from build123d import *

# Parameters (mm, degrees)
SKETCH1_R           = 60
BOSS_EXTRUDE1_DEPTH = 1500
CUT_EXTRUDE1_REACH  = 1504.398


with BuildPart() as part:
    # Sketch1 → Boss-Extrude1 (new body)
    with BuildSketch(Plane(origin=(0, 0, 0), x_dir=(1, 0, 0), z_dir=(0, 1, 0))):
        with Locations(Location((0, 0, 0), (0, 0, 270))):
            Circle(SKETCH1_R)
    extrude(amount=BOSS_EXTRUDE1_DEPTH)

    # Sketch2 → Cut-Extrude1 (cut, up to next)
    with BuildSketch(Plane(origin=(0, 1500, 0), x_dir=(1, 0, 0), z_dir=(0, 1, 0)), mode=Mode.PRIVATE) as cut_extrude1_sk1:
        Polygon((-10.998522628, 19.05), (-21.997045256, 0), (-10.998522628, -19.05), (10.998522628, -19.05), (21.997045256, 0), (10.998522628, 19.05), align=None)
    cut_extrude1_tool1 = extrude(cut_extrude1_sk1.sketch, amount=-CUT_EXTRUDE1_REACH, mode=Mode.PRIVATE) & part.part
    add(cut_extrude1_tool1.solids().sort_by_distance((0, 1500, 0))[0], mode=Mode.SUBTRACT)


solid = part.part
Verification items for the finished model (mm, model axes). Round coordinates to 2 decimals unless told otherwise and drop trailing zeros. Loops run counter-clockwise (first coordinate to the right, second up) from the corner with the lowest first, then second, coordinate; pieces in that order, holes last. Notation, with made-up numbers: (23, 67.25) - (36, 67.25) arc R27 cw to (36, 88.25) - close; hole circle Ø10 at (63.25, 4.5). An arc over 180 degrees is marked (long way). Use one line per item in the form item = value.
1. Gauge pin test, flat ends, axial feed: pin 1 Ø3 at (x, y) = (21, 974) entering from -Z; pin 2 Ø4 at (y, z) = (670.5, 43.5) entering from +X; pin 3 Ø3 at (y, z) = (866.5, 30) entering from +X. Record the tip position at first contact, or that the pin passes through.
A:
pin_1 = -56.74
pin_2 = 43.33
pin_3 = 52.8
2. Section check B-B on x = -36. Record the cut outline in (y, z), and give its area (3 significant figures).
A:
outline = (0, -48) - (1500, -48) - (1500, 48) - (0, 48) - close
area = 144,000 mm²
3. Section check A-A on y = 752.5. Record the cut outline in (x, z), and give its area (3 significant figures).
A:
outline = circle Ø120 at (0, 0); hole (-22, 0) - (-11, -19.05) - (11, -19.05) - (22, 0) - (11, 19.05) - (-11, 19.05) - close
area = 10,100 mm²
4. Scan lines: probe 1 along Z at (x, y) = (-4, 234.5); probe 2 along X at (y, z) = (947.5, 1); probe 3 along Z at (x, y) = (11.5, 609.5). Record each from-to range of solid material in increasing order.
A:
probe_1 = -59.87 to -19.05, 19.05 to 59.87
probe_2 = -59.99 to -21.42, 21.42 to 59.99
probe_3 = -58.89 to -18.18, 18.18 to 58.89
